Design review of the part built by this model. Coordinates are the model's own, in mm. A direction names the side the tool comes from. Give positions to 0.01 mm unless a question says otherwise; leave off trailing zeros. Loops run counter-clockwise (first coordinate to the right, second up) from the corner with the lowest first, then second, coordinate; pieces in that order, holes last. Notation, with made-up numbers: M 76,-37 L 123,-37 A15 cw 123,-19 Z; hole C 2.25,57.5 d7. An arc over 180 degrees is marked long. Use CSV: the item, a comma, the result in double quotes.
from build123d import *

# Parameters (mm, degrees)
CROQUIS2_R                 = 12.7
SALIENTE_EXTRUIR1_DEPTH    = 25.4
CORTAR_EXTRUIR1_DEPTH      = 185.585264851
CORTAR_EXTRUIR1_DEPTH_BACK = 76.2
CROQUIS7_W                 = 76.2
CROQUIS7_H                 = 12.7
SALIENTE_EXTRUIR2_DEPTH    = 25.4
REDONDEO1_R                = 5.08


with BuildPart() as part:
    # Croquis2 → Saliente-Extruir1 (new body)
    with BuildSketch(Plane(origin=(0, 0, 0), x_dir=(1, 0, 0), z_dir=(0, 1, 0))):
        with BuildLine():
            Line((139.3, -50.8), (-139.3, -50.8))
            ThreePointArc((-139.3, -50.8), (-148.280256121, -47.080256121), (-152, -38.1))
            Line((-152, -38.1), (-152, 38.1))
            ThreePointArc((-152, 38.1), (-148.280256121, 47.080256121), (-139.3, 50.8))
            Line((-139.3, 50.8), (139.3, 50.8))
            ThreePointArc((139.3, 50.8), (148.280256121, 47.080256121), (152, 38.1))
            Line((152, 38.1), (152, -38.1))
            ThreePointArc((152, -38.1), (148.280256121, -47.080256121), (139.3, -50.8))
        make_face()
        with Locations(Location((-126.6, 0, 0), (0, 0, 270))):
            Circle(CROQUIS2_R, mode=Mode.SUBTRACT)
        with Locations(Location((126.6, 0, 0), (0, 0, 270))):
            Circle(CROQUIS2_R, mode=Mode.SUBTRACT)
    extrude(amount=SALIENTE_EXTRUIR1_DEPTH)

    # Croquis7 → Cortar-Extruir1 (cut, two sides: drawn at the far end of the back side and taken through both)
    with BuildSketch(Plane(origin=(0, 0, -50.8), x_dir=(-1, 0, 0), z_dir=(0, 0, -1)).offset(-CORTAR_EXTRUIR1_DEPTH_BACK)):
        with Locations((0, 6.35)):
            Rectangle(CROQUIS7_W, CROQUIS7_H)
    extrude(amount=CORTAR_EXTRUIR1_DEPTH + CORTAR_EXTRUIR1_DEPTH_BACK, mode=Mode.SUBTRACT)

    # Croquis9 → Saliente-Extruir2 (add)
    with BuildSketch(Plane(origin=(0, 0, -50.8), x_dir=(-1, 0, 0), z_dir=(0, 0, -1))):
        with BuildLine():
            Line((-37.968696545, 101.6), (-37.968696545, 25.4))
            Line((-37.968696545, 25.4), (38.231303455, 25.4))
            Line((38.231303455, 25.4), (38.231303455, 101.6))
            ThreePointArc((38.231303455, 101.6), (0.131303455, 139.7), (-37.968696545, 101.6))
        make_face()
    extrude(amount=-SALIENTE_EXTRUIR2_DEPTH)

    # Croquis11 → Refrentado para tornillo con cabeza troncocónica de 9/162 (revolve, cut)
    with BuildSketch(Plane(origin=(0, 101.965288162, -50.8), x_dir=(0, 1, 0), z_dir=(1, 0, 0))):
        Polygon((0, 0), (0, 101.6), (7.53999, 101.6), (7.53999, 9.9314), (13.69187, 9.9314), (13.69187, 0.635), (14.32687, 0), align=None)
    revolve(axis=Axis((0, 101.965288162, -57.15), (0, 0, 1)), mode=Mode.SUBTRACT)

    # Redondeo1
    redondeo1_edges = [part.edges().sort_by_distance(p)[0] for p in [
        (148.280256121, 25.4, -47.080256121),
        (88.634348272, 25.4, -50.8),
        (-148.280256121, 25.4, -47.080256121),
        (-152, 25.4, 0),
        (-148.280256121, 25.4, 47.080256121),
        (0, 25.4, 50.8),
        (-88.765651728, 25.4, -50.8),
        (-38.231303455, 63.5, -25.4),
        (-0.131303455, 25.4, -25.4),
        (-38.231303455, 25.4, -38.1),
        (37.968696545, 63.5, -25.4),
        (37.968696545, 25.4, -38.1),
        (-0.131303455, 139.7, -25.4),
        (-38.231303455, 63.5, -50.8),
        (-0.131303455, 139.7, -50.8),
        (37.968696545, 63.5, -50.8),
        (148.280256121, 25.4, 47.080256121),
        (152, 25.4, 0),
    ]]
    fillet(redondeo1_edges, radius=REDONDEO1_R)


solid = part.part
(1) We need section C-C on z = 28.5. State the section outline as (x, y) points.
A:
outline,"M -152,0 L 152,0 L 152,20.32 A5.08 ccw 146.92,25.4 L -146.92,25.4 A5.08 ccw -152,20.32 Z"
(2) The part is to be moulded in two halves that separate along Y. For faces 1 (the flat face through (2, 10, 50.8)), 2 (the flat face through (2, 0, 33)), 3 (the cylindrical face through (-0.97, 139.69, -38.21)), 4 (the cylindrical face through (2.89, 108.93, -33.24)), say which applies: released by +Y, released by -Y, zero draft, split by the parting line, or undercut.
A:
face 1,"zero draft"
face 2,"released by -Y"
face 3,"released by +Y"
face 4,"undercut"
(3) Wall thickness on line 1 along X through (y, z) = (10.5, 0); line 2 along X through (y, z) = (17.75, 0); line 3 along X through (y, z) = (23, -11): over which ranges is each line inside the solid? List them lowest first. Write a range as [from, to].
A:
line 1,"[-152, -139.3], [-113.9, -38.1], [38.1, 113.9], [139.3, 152]"
line 2,"[-152, -139.3], [-113.9, 113.9], [139.3, 152]"
line 3,"[-151.24, -132.95], [-120.25, 120.25], [132.95, 151.24]"
(4) Machinability: for faces 5 (the cylindrical face through (137.309, 12.522, 6.827)), 6 (the flat face through (37.969, 67, -38)), 7 (the flat face through (2, 25.4, -1)), 8 (the cylindrical face through (-148.38, 10.02, -46.98)), 9 (the flat face through (1, 6, 25.4)), which of the approach directions +Z, -Z, +X, -X, +Y, -Y give a long, thin tool a straight path to every point of the face, cutting with its end or side? Answer none if there is none.
A:
face 5,"+Y, -Y"
face 6,"+Z, -Z, +X, +Y"
face 7,"+Z, +Y"
face 8,"-Z, -X, +Y, -Y"
face 9,"-Z, -Y"
(5) Clearance check with flat-ended pins moving along their axes: P1, Ø4, axis at x = 100.5, z = -19.5, coming from the +Y side; P2, Ø4, axis at x = 13.5, y = 6.5, coming from the -Z side; P3, Ø17, axis at y = 51, z = -34.5, coming from the +X side; P4, Ø23, axis at x = -126.6, z = 0, coming from the +Y side. State where each tip first meets the part, or that it passes through.
A:
P1,"y = 25.4"
P2,"z = 25.4"
P3,"x = 37.97"
P4,"through"
(6) We need section B-B on x = 126.6. State the section outline as (y, z) points.
A:
outline,"M 0,-50.8 L 20.32,-50.8 A5.08 ccw 25.4,-45.72 L 25.4,-12.7 L 0,-12.7 Z; M 0,12.7 L 25.4,12.7 L 25.4,45.72 A5.08 ccw 20.32,50.8 L 0,50.8 Z"
(7) We need section A-A on z = 0. State the section outline as (x, y) points.
A:
outline,"M -152,0 L -139.3,0 L -139.3,25.4 L -146.92,25.4 A5.08 ccw -152,20.32 Z; M -113.9,0 L -38.1,0 L -38.1,12.7 L 38.1,12.7 L 38.1,0 L 113.9,0 L 113.9,25.4 L -113.9,25.4 Z; M 139.3,0 L 152,0 L 152,20.32 A5.08 ccw 146.92,25.4 L 139.3,25.4 Z"
(8) We need section D-D on y = 79. State the section outline as (x, z) points, then the cut area to 3 significant figures.
A:
outline,"M -38.23,-45.72 A5.08 ccw -33.15,-50.8 L 32.89,-50.8 A5.08 ccw 37.97,-45.72 L 37.97,-30.48 A5.08 ccw 32.89,-25.4 L -33.15,-25.4 A5.08 ccw -38.23,-30.48 Z"
area,"1,910 mm²"
